Source: three-view drawing plus pictorial views. Frame: mm from the lowest corner of the part. A direction names the side the tool comes from. Give positions to 0.01 mm unless a question says otherwise; leave off trailing zeros. Write each loop counter-clockwise with the first axis right and the second up, starting at its lowest first coordinate (ties: lowest second). Pieces come first, ordered by that corner, then holes.
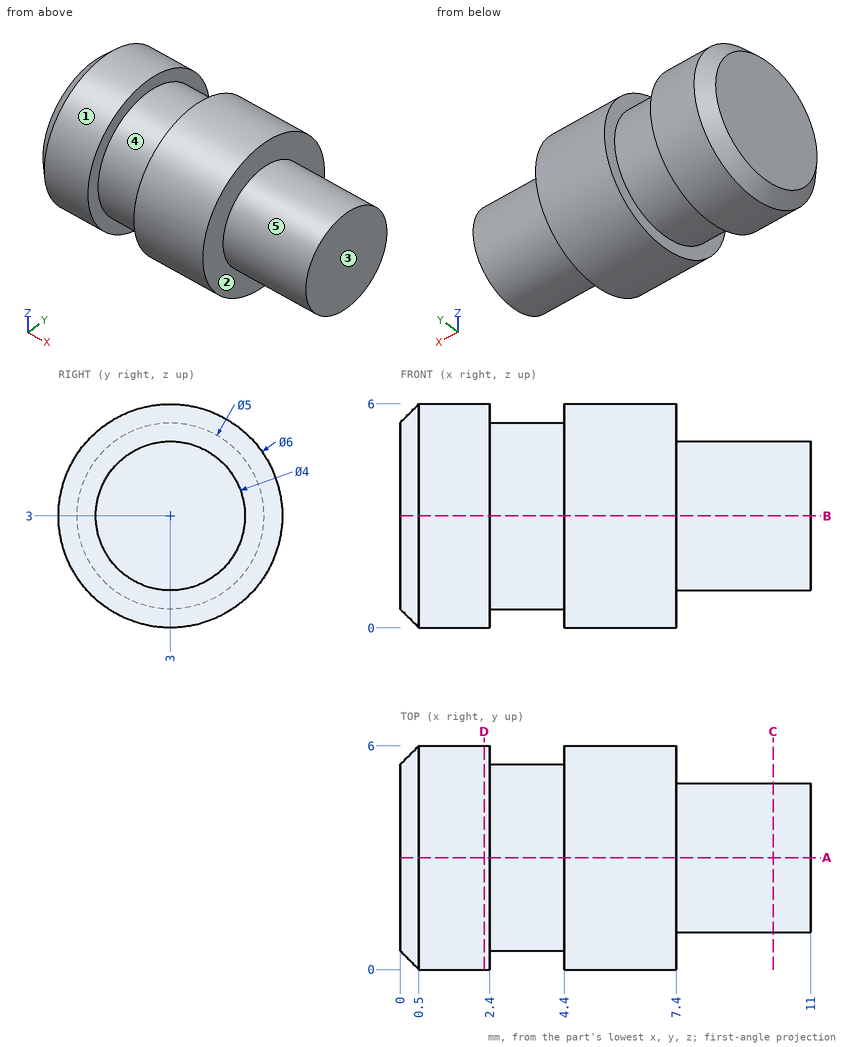
Q1. Pull-direction query (X, two-part tool) for the marked faces 3, 4 and 5; classes: released by +X, released by -X, zero draft, split by the parting line, or undercut.
Filled sheet:
face 3: released by +X
face 4: undercut
face 5: zero draft
Q2. Ray query, line 1 along X through (y, z) = (1.5, 4.85); line 2 along X through (y, z) = (0.7, 4.7); line 3 along Y through (x, z) = (2.75, 1.6). Return the intervals inside material, ascending.
Filled sheet:
line 1: x = 0 to 7.4
line 2: x = 0.36 to 2.4, 4.4 to 7.4
line 3: y = 0.93 to 5.07
Q3. Section D-D on x = 2.25. Output: boundary loops of the cut face in (y, z), plus the area to 3 significant figures.
Filled sheet:
outline: circle Ø6 at (3, 3)
area: 28.3 mm2
Q4. Pin query (flat end, axial travel): P1, Ø2, axis at x = 9, z = 3.5, coming from the -Y side. Return the tip coordinate at first contact, or that it passes through.
Filled sheet:
P1: stops at y = 1
Q5. Section A-A on y = 3. Output: boundary loops of the cut face in (x, z).
Filled sheet:
outline: (0, 0.5) - (0.5, 0) - (2.4, 0) - (2.4, 0.5) - (4.4, 0.5) - (4.4, 0) - (7.4, 0) - (7.4, 1) - (11, 1) - (11, 5) - (7.4, 5) - (7.4, 6) - (4.4, 6) - (4.4, 5.5) - (2.4, 5.5) - (2.4, 6) - (0.5, 6) - (0, 5.5) - close
Q6. Access query for the marked faces 1 and 2. Directions: +Z, -Z, +X, -X, +Y, -Y. A direction counts if a zero-diameter tool reaches every point of the face in a straight line with its end or side. Return the directions, or none.
Filled sheet:
face 1: +X, -X
face 2: +X
Q7. Section C-C on x = 10. Output: boundary loops of the cut face in (y, z).
Filled sheet:
outline: circle Ø4 at (3, 3)
